The listing builds one solid part. Answer for the finished solid, in the listing's coordinates (mm). Round coordinates to 2 decimals unless told otherwise and drop trailing zeros. Order: outer loops, then holes, each group sorted by start corner. A loop starts at its lowest first (then second) coordinate and runs counter-clockwise, first axis right, second up. Notation, with made-up numbers: (29.5, 16.25) - (77.5, 16.25) arc R8 ccw to (77.5, 29.25) - close; hole circle Ø10 at (0, 1). An arc over 180 degrees is marked (long way). One line per item, written item: value. Start each with the question number.
1. Flat-ended cylindrical pins translate along their axes: P1, Ø3, axis at x = 55, z = -10.5, coming from the -Y side; P2, Ø3, axis at x = 90, y = -6, coming from the +Z side; P3, Ø8, axis at x = 48.5, y = 0.5, coming from the -Z side. Find the tip coordinate at first contact, or state that the pin passes through.
2. For a pull along X with two mould halves and no side action, classify faces 1 (the cylindrical face through (107.62, -5.85, -11.13)), 2 (the flat face through (0, 0, 0)), 3 (the flat face through (115.78, -0.09, -27)) as released by +X, released by -X, zero draft, split by the parting line, or undercut.
3. Straight lines are drawn through the part: line 1 (Z direction, x = 80.5, y = -0.25); line 2 (X direction, y = -2.25, z = -1); line 3 (Z direction, x = 110, y = 3.75). For each, find the intervals that lie inside material, in ascending order.
4. Section A-A, the plane x = 68 is taken. Give the vertices of the cut face in (y, z) (1 decimal).
from build123d import *

# Parameters (mm, degrees)
F1_R     = 7.9375
F4_D     = 3.175
F4_DEPTH = 7.9385001
F5_D     = 3.175
F6_SIZE  = 1.5875


with BuildPart() as f2:
    # F2: sweep along a path in F0
    with BuildLine(Plane.XZ) as f2_path:
        Line((0, 0), (83.6394877579, 0))
        ThreePointArc((83.6394877579, 0), (88.4995673489, -0.9667299371), (92.6197438789, -3.7197438789))
        Line((92.6197438789, -3.7197438789), (115.8407683632, -26.9407683632))
    # F1 (on Right) → F2 (sweep)
    with BuildSketch(Plane.YZ):
        Circle(F1_R)
    sweep(path=f2_path.line)

    # F4 (through all, one way)
    with BuildSketch(Plane.XZ):
        with Locations((9.525, 0)):
            Circle(F4_D / 2)
    extrude(amount=-F4_DEPTH, mode=Mode.SUBTRACT)

    # F5 (through all)
    with Locations(Plane(origin=(0, 0, 0), x_dir=(1, 0, 0), z_dir=(0, 1, 0))):
        with Locations((9.525, 0)):
            Hole(F5_D / 2)

    # F6
    f6_edges = [f2.edges().sort_by_distance(p)[0] for p in [
        (0, -7.9375, 0),
        (115.840768, -7.9375, -26.940768),
    ]]
    chamfer(f6_edges, length=F6_SIZE)


solid = f2.part
Answer list:
1. P1: passes through
1. P2: stops at z = 5.56
1. P3: stops at z = -7.94
2. face 1: split by the parting line
2. face 2: released by -X
2. face 3: released by +X
3. line 1: z = -7.93 to 7.93
3. line 2: x = 0 to 8.29, 10.76 to 100.66
3. line 3: z = -30.75 to -11.21
4. outline: circle Ø15.9 at (0, 0)
